Design review of the part built by this model. Coordinates are the model's own, in mm. A direction names the side the tool comes from. Coordinates: 2 decimals unless noted, no trailing zeros. Loops run counter-clockwise (first coordinate to the right, second up) from the corner with the lowest first, then second, coordinate; pieces in that order, holes last. Notation, with made-up numbers: (10.5, 5) -> (29.5, 5) arc R6 ccw to (29.5, 14) -> close; hole circle Ø4 at (-3.75, 12). An arc over 180 degrees is marked (long way). Use a Markdown table: item, result. Add a question column.
Q1. For faces 4 (the face through (3, 0, 0)), 5 (the face through (1.15, 0.07, 10)), list the 3-axis set-ups (+Z, -Z, +X, -X, +Y, -Y) from which the entire face can be reached by the end or side of a thin tool; tool diameter is ignored.
Q2. Take a section at A-A on y = 0. Write out the cut boundary in (x, z), plus the area to 3 significant figures.
Q3. Take a section at B-B on x = 0. Write out the cut boundary in (y, z).
Q4. Take a section at C-C on z = 3.25. Write out the cut boundary in (x, y).
Q5. For probe 1 along Y at (x, z) = (0, 16.5); probe 2 along Z at (x, y) = (-1.5, -1); probe 3 along X at (y, z) = (-1.75, 1.75), list the stretches that pass through material, from the lowest coordinate up.
Q6. Take a section at D-D on z = 16.75. Write out the cut boundary in (x, y), plus the area to 3 significant figures.
Q7. Draft analysis for pull direction X (two halves, no side actions). For faces 1 (the face through (-3, 0, 0)), 2 (the face through (2.5, 0, 5)), 3 (the face through (-0.651, 4.957, 12.082)), state which applies: pulls with the +X half, pulls with the -X half, needs draft (parallel to the pull), parting line crosses it, or undercut.
Q8. Clearance check with flat-ended pins moving along their axes: pin 1 Ø6 at (y, z) = (-3.5, 7) entering from -X; pin 2 Ø3 at (x, z) = (-4, 17) entering from +Y; pin 3 Ø1.6 at (x, y) = (0, 0) entering from -Z; pin 4 Ø2.5 at (x, y) = (1, -1.5) entering from -Z. State where each tip first meets the part, or that it passes through.
from build123d import *

# Parameters (mm, degrees)
CROQUIS1_R              = 5
SALIENTE_EXTRUIR1_DEPTH = 20
CROQUIS3_W              = 5
CROQUIS3_H              = 10
CORTAR_EXTRUIR1_DEPTH   = 10
CROQUIS4_R              = 1
CORTAR_EXTRUIR2_DEPTH   = 10


with BuildPart() as part:
    # Croquis1 → Saliente-Extruir1 (new body)
    with BuildSketch(Plane.XY):
        Circle(CROQUIS1_R)
    extrude(amount=SALIENTE_EXTRUIR1_DEPTH)

    # Croquis3 → Cortar-Extruir1 (cut)
    with BuildSketch(Plane(origin=(0, 0, 0), x_dir=(-1, 0, 0), z_dir=(0, 0, -1))):
        Rectangle(CROQUIS3_W, CROQUIS3_H)
    extrude(amount=-CORTAR_EXTRUIR1_DEPTH, mode=Mode.SUBTRACT)

    # Croquis4 → Cortar-Extruir2 (cut)
    with BuildSketch(Plane(origin=(2.5, -4.330127019, 10), x_dir=(-1, 0, 0), z_dir=(0, 0, -1))):
        with Locations((2.5, 4.330127019)):
            Circle(CROQUIS4_R)
    extrude(amount=-CORTAR_EXTRUIR2_DEPTH, mode=Mode.SUBTRACT)


solid = part.part
Answer list:
| question | item | result |
|---|---|---|
| 1 | face 4 | -Z, +X, -X, +Y, -Y |
| 1 | face 5 | -Z, +Y, -Y |
| 2 | outline | (-5, 0) -> (-2.5, 0) -> (-2.5, 10) -> (-1, 10) -> (-1, 20) -> (-5, 20) -> close; (1, 10) -> (2.5, 10) -> (2.5, 0) -> (5, 0) -> (5, 20) -> (1, 20) -> close |
| 2 | area | 130 mm² |
| 3 | outline | (-5, 10) -> (-1, 10) -> (-1, 20) -> (-5, 20) -> close; (1, 10) -> (5, 10) -> (5, 20) -> (1, 20) -> close |
| 4 | outline | (-2.5, -4.33) -> (-2.5, 4.33) arc R5 ccw to start; (2.5, -4.33) arc R5 ccw to (2.5, 4.33) -> close |
| 5 | probe 1 | -5 to -1, 1 to 5 |
| 5 | probe 2 | 10 to 20 |
| 5 | probe 3 | -4.68 to -2.5, 2.5 to 4.68 |
| 6 | outline | circle Ø10 at (0, 0); hole circle Ø2 at (0, 0) |
| 6 | area | 75.4 mm² |
| 7 | face 1 | needs draft |
| 7 | face 2 | undercut |
| 7 | face 3 | parting line crosses it |
| 8 | pin 1 | x = -4.97 |
| 8 | pin 2 | y = 4.33 |
| 8 | pin 3 | through |
| 8 | pin 4 | z = 10 |
